```python
from build123d import *

# Parameters (mm, degrees)
SKETCH_1_W          = 210
SKETCH_1_H          = 50
EXTRUDE_1_DEPTH     = 5
SKETCH_3_R          = 2.25
CUT_EXTRUDE_1_DEPTH = 5
SKETCH_4_W          = 210
SKETCH_4_H          = 5
EXTRUDE_2_DEPTH     = 61
CUT_EXTRUDE_2_REACH = 227.734
SKETCH_6_W          = 60
SKETCH_6_H          = 5
FILLET_1_R          = 10
CUT_EXTRUDE_3_REACH = 227.734
SKETCH_7_W          = 88
SKETCH_7_H          = 5
FILLET_2_R          = 10
FILLET_6_R          = 3
SKETCH_11_R         = 2.25
CUT_EXTRUDE_4_DEPTH = 225.67977212


with BuildPart() as part:
    # 草图1 → 凸台-拉伸1 (new body)
    with BuildSketch(Plane.XY):
        with Locations((105, 25)):
            Rectangle(SKETCH_1_W, SKETCH_1_H)
    extrude(amount=EXTRUDE_1_DEPTH)

    # 草图3 → 切除-拉伸1 (cut)
    with BuildSketch(Plane.XY.offset(5)):
        with Locations((157.25, 25)):
            Circle(SKETCH_3_R)
        with Locations((187.25, 25)):
            Circle(SKETCH_3_R)
        with Locations(Location((22.75, 25, 0), (0, 0, 180))):
            Circle(SKETCH_3_R)
        with Locations(Location((52.75, 25, 0), (0, 0, 180))):
            Circle(SKETCH_3_R)
    extrude(amount=-CUT_EXTRUDE_1_DEPTH, mode=Mode.SUBTRACT)

    # 草图4 → 凸台-拉伸2 (add)
    with BuildSketch(Plane.XY.offset(5)):
        with Locations((105, 2.5)):
            Rectangle(SKETCH_4_W, SKETCH_4_H)
    extrude(amount=EXTRUDE_2_DEPTH)

    # 草图6 → 切除-拉伸2 (cut, up to next)
    with BuildSketch(Plane.XY.offset(66), mode=Mode.PRIVATE) as cut_extrude_2_sk1:
        with Locations((180, 2.5)):
            Rectangle(SKETCH_6_W, SKETCH_6_H)
    cut_extrude_2_tool1 = extrude(cut_extrude_2_sk1.sketch, amount=-CUT_EXTRUDE_2_REACH, mode=Mode.PRIVATE) & part.part
    add(cut_extrude_2_tool1.solids().sort_by_distance((180, 2.5, 66))[0], mode=Mode.SUBTRACT)

    # 圆角1
    # the kernel refuses this fillet: 10 mm, written as the material it adds along each edge
    with BuildSketch(Plane(origin=(150, 5, 0), x_dir=(0, -1, 0), z_dir=(0, 0, 1))) as fillet_1_piece_1:
        with BuildLine():
            CenterArc((10, 8.660254038), FILLET_1_R, 180, 60)
            Line((0, 8.660254038), (0, 0))
            Line((0, 0), (5, 0))
        make_face()
    extrude(amount=5)

    # 草图7 → 切除-拉伸3 (cut, up to next)
    with BuildSketch(Plane.XY.offset(66), mode=Mode.PRIVATE) as cut_extrude_3_sk1:
        with Locations((44, 2.5)):
            Rectangle(SKETCH_7_W, SKETCH_7_H)
    cut_extrude_3_tool1 = extrude(cut_extrude_3_sk1.sketch, amount=-CUT_EXTRUDE_3_REACH, mode=Mode.PRIVATE) & part.part
    add(cut_extrude_3_tool1.solids().sort_by_distance((44, 2.5, 66))[0], mode=Mode.SUBTRACT)

    # 圆角2
    # the kernel refuses this fillet: 10 mm, written as the material it adds along each edge
    with BuildSketch(Plane(origin=(88, 5, 0), x_dir=(0, -1, 0), z_dir=(0, 0, 1))) as fillet_2_piece_1:
        with BuildLine():
            CenterArc((10, -8.660254038), FILLET_2_R, 120, 60)
            Line((0, -8.660254038), (0, 0))
            Line((0, 0), (5, 0))
        make_face()
    extrude(amount=5)

    # 圆角6
    # the kernel refuses this fillet: 3 mm, written as the material it adds along each edge
    with BuildSketch(Plane(origin=(150, 5, 5), x_dir=(1, 0, 0), z_dir=(0, -1, 0))) as fillet_6_piece_1_section:
        with BuildLine():
            CenterArc((FILLET_6_R, FILLET_6_R), FILLET_6_R, 180, 90)
            Line((0, FILLET_6_R), (0, 0))
            Line((0, 0), (FILLET_6_R, 0))
        make_face()
    fillet_6_piece_1 = extrude(amount=5, mode=Mode.PRIVATE)
    fillet_6_piece_1 = fillet_6_piece_1 - Plane(origin=(158.660254038, -5, 5.756133445), x_dir=(0, -1, 0), z_dir=(0, 0, -1)) * Cylinder(10, 22, mode=Mode.PRIVATE)
    add(fillet_6_piece_1)
    with BuildSketch(Plane(origin=(88, 5, 5), x_dir=(-1, 0, 0), z_dir=(0, -1, 0))) as fillet_6_piece_2_section:
        with BuildLine():
            CenterArc((FILLET_6_R, -FILLET_6_R), FILLET_6_R, 90, 90)
            Line((0, -FILLET_6_R), (0, 0))
            Line((0, 0), (FILLET_6_R, 0))
        make_face()
    fillet_6_piece_2 = extrude(amount=5, mode=Mode.PRIVATE)
    fillet_6_piece_2 = fillet_6_piece_2 - Plane(origin=(79.339745962, -5, 5.756136784), x_dir=(0, -1, 0), z_dir=(0, 0, -1)) * Cylinder(10, 22, mode=Mode.PRIVATE)
    add(fillet_6_piece_2)

    # 草图11 → 切除-拉伸4 (cut, through all)
    with BuildSketch(Plane(origin=(0, 5, 0), x_dir=(1, 0, 0), z_dir=(0, 1, 0))):
        with Locations(Location((98.991167509, -29.5, 0), (0, 0, 180))):
            Circle(SKETCH_11_R)
        with Locations(Location((138.991167509, -29.5, 0), (0, 0, 180))):
            Circle(SKETCH_11_R)
        with Locations(Location((98.991167509, -41.5, 0), (0, 0, 180))):
            Circle(SKETCH_11_R)
        with Locations(Location((138.991167509, -41.5, 0), (0, 0, 180))):
            Circle(SKETCH_11_R)
    extrude(amount=-CUT_EXTRUDE_4_DEPTH, mode=Mode.SUBTRACT)


solid = part.part
```
Input: part model. Units: mm. Frame: model coordinates. A direction names the side the tool comes from. Give positions to 0.01 mm unless a question says otherwise; leave off trailing zeros. Loops run counter-clockwise (first coordinate to the right, second up) from the corner with the lowest first, then second, coordinate; pieces in that order, holes last.
1) Section query B-B on z = 29.5. Return the cut outline in (x, y), and give its area (3 significant figures).
A:
outline: (88, 0) - (96.74, 0) - (96.74, 5) - (88, 5) - close; (101.24, 0) - (136.74, 0) - (136.74, 5) - (101.24, 5) - close; (141.24, 0) - (150, 0) - (150, 5) - (141.24, 5) - close
area: 265 mm2
2) Line query: L1, parallel to Z at x = 81, y = 19; L2, parallel to Y at x = 52, z = 1. Output: solid intervals per line, ascending.
A:
L1: z = 0 to 5
L2: y = 5 to 22.88, 27.12 to 50
3) Section query A-A on x = 52.75. Return the cut outline in (y, z).
A:
outline: (5, 0) - (22.75, 0) - (22.75, 5) - (5, 5) - close; (27.25, 0) - (50, 0) - (50, 5) - (27.25, 5) - close
4) Reachability of faces 4 (the flat face through (184, 5, 3)), 5 (the flat face through (88, 2, 37)), 6 (the flat face through (39, 5, 3)), 7 (the flat face through (150, 2, 37)), 8 (the flat face through (106, 26, 5)) from +Z, -Z, +X, -X, +Y, -Y: full face, straight path, thin tool, end or side. Return the list, or none.
A:
face 4: +Z, -Z, +X, -Y
face 5: +Z, -X, +Y, -Y
face 6: +Z, -Z, -X, -Y
face 7: +Z, +X, +Y, -Y
face 8: +Z, +X, -X, +Y
5) Section query C-C on y = 25. Return the cut outline in (x, z), and give its area (3 significant figures).
A:
outline: (0, 0) - (20.5, 0) - (20.5, 5) - (0, 5) - close; (25, 0) - (50.5, 0) - (50.5, 5) - (25, 5) - close; (55, 0) - (155, 0) - (155, 5) - (55, 5) - close; (159.5, 0) - (185, 0) - (185, 5) - (159.5, 5) - close; (189.5, 0) - (210, 0) - (210, 5) - (189.5, 5) - close
area: 960 mm2
6) Mould query, pull axis Y, two halves, no side actions, for faces 1 (the flat face through (119, 5, 35)), 2 (the cylindrical face through (189.33, 24.14, 2.54)), 3 (the cylindrical face through (101.24, 2.54, 29.6)). Classes: released by +Y, released by -Y, zero draft, split by the parting line, or undercut.
A:
face 1: released by +Y
face 2: undercut
face 3: zero draft
7) Contact query for flat-ended pins moving along their axis: pin 1 (5.5 mm diameter, centred on x = 21, z = 2.5, fed in from -Y); pin 2 (1.5 mm diameter, centred on y = 1.5, z = 41, fed in from +X); pin 3 (1.5 mm diameter, centred on y = 2.5, z = 28.5, fed in from -X). Output: stop coordinate, or through.
A:
pin 1: stops at y = 5
pin 2: stops at x = 150
pin 3: stops at x = 88
8) Section query D-D on z = 15. Return the cut outline in (x, y).
A:
outline: (88, 0) - (150, 0) - (150, 5) - (88, 5) - close
